Job drawing, mm, ordinate dimensions from the low corner. One solid piece. Give positions to 0.01 mm unless a question says otherwise; leave off trailing zeros. Write each loop counter-clockwise with the first axis right and the second up, starting at its lowest first coordinate (ties: lowest second). Pieces come first, ordered by that corner, then holes. Notation, with made-up numbers: M 64.25,10.25 L 104.25,10.25 A26 cw 104.25,48.25 Z; hole C 29.5,10.5 d3. An arc over 180 degrees is marked long. Answer as CSV lines item,"result". Start each with the question number.
1) Slice it at D-D, the plane y = 4.5. Give the cut face in (x, z).
2) Slice it at B-B, the plane y = 18. Give the cut face in (x, z) (3 decimals), plus the area to 3 significant figures.
3) Pin check, flat tips, straight feed: pin 1 Ø3.5 at (x, y) = (31.875, 18) entering from +Z; pin 2 Ø2 at (x, y) = (12.25, 12.25) entering from -Z; pin 3 Ø3 at (x, z) = (11, 1) entering from +Y. Stop position of each tip, or through.
4) Wall check: line 1 along X through (y, z) = (18, 1.2) (3 decimals); line 2 along X through (y, z) = (25, 1.1); line 3 along X through (y, z) = (23.75, 3.8). Give the ranges that are in metal, low to high. Write a range as from..to.
5) Slice it at A-A, the plane z = 2.3. Give the cut face in (x, y) (3 decimals), plus the area to 3 significant figures.
6) Slice it at C-C, the plane x = 18. Give the cut face in (y, z), plus the area to 3 significant figures.
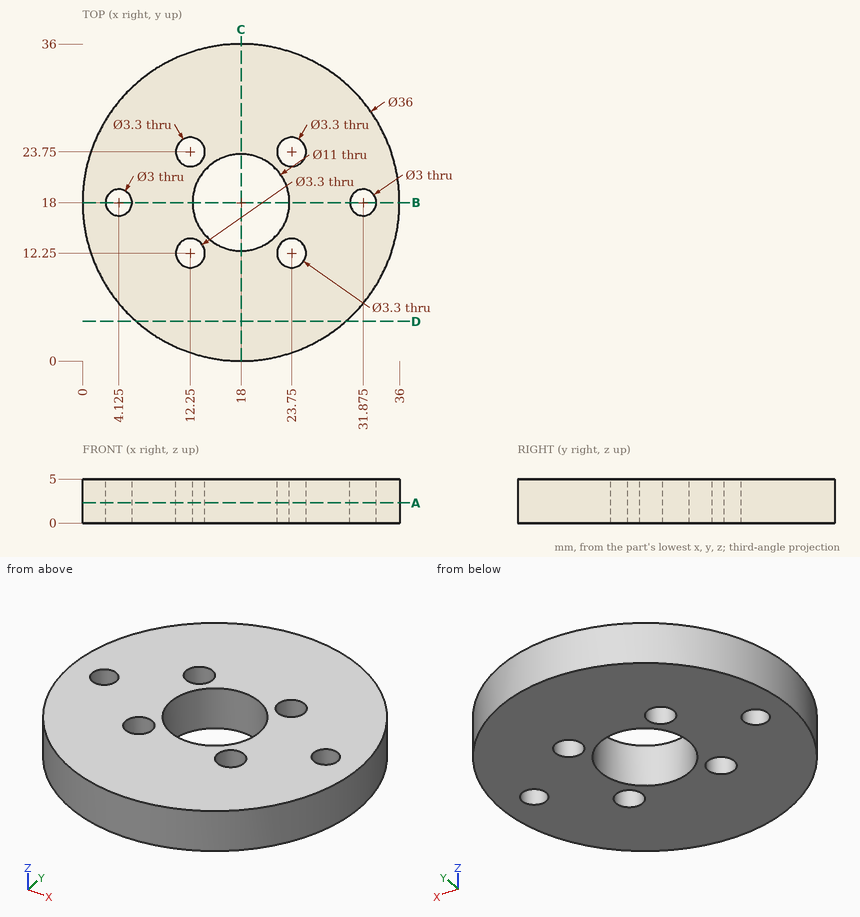
Found:
1,outline,"M 6.09,0 L 29.91,0 L 29.91,5 L 6.09,5 Z"
2,outline,"M 0,0 L 2.625,0 L 2.625,5 L 0,5 Z; M 5.625,0 L 12.5,0 L 12.5,5 L 5.625,5 Z; M 23.5,0 L 30.375,0 L 30.375,5 L 23.5,5 Z; M 33.375,0 L 36,0 L 36,5 L 33.375,5 Z"
2,area,"95.0 mm²"
3,pin 1,"z = 5"
3,pin 2,"through"
3,pin 3,"y = 35.14"
4,line 1,"0..2.625, 5.625..12.5, 23.5..30.375, 33.375..36"
4,line 2,"1.42..11.17, 13.33..22.67, 24.83..34.58"
4,line 3,"0.94..10.6, 13.9..22.1, 25.4..35.06"
5,outline,"C 18,18 d36; hole C 4.125,18 d3; hole C 12.25,12.25 d3.3; hole C 12.25,23.75 d3.3; hole C 18,18 d11; hole C 23.75,12.25 d3.3; hole C 23.75,23.75 d3.3; hole C 31.875,18 d3"
5,area,"874 mm²"
6,outline,"M 0,0 L 12.5,0 L 12.5,5 L 0,5 Z; M 23.5,0 L 36,0 L 36,5 L 23.5,5 Z"
6,area,"125 mm²"
